from build123d import *

# Parameters (mm, degrees)
SKETCH1_R           = 55.5
BOSS_EXTRUDE1_DEPTH = 29.4
CUT_EXTRUDE1_DEPTH  = 19.4
SKETCH3_R           = 1.65
SKETCH3_R_2         = 2.8
CUT_EXTRUDE2_DEPTH  = 133.783969288
SKETCH4_R           = 11.3
CUT_EXTRUDE3_DEPTH  = 2
SKETCH5_R           = 3.3
CUT_EXTRUDE4_DEPTH  = 5
SKETCH6_R           = 40.3
SKETCH6_R_2         = 30.3
BOSS_EXTRUDE2_DEPTH = 59.8
BOSS_EXTRUDE3_DEPTH = 119.6
BOSS_EXTRUDE4_START = -29.4
BOSS_EXTRUDE4_DEPTH = 29.4
FILLET1_R           = 10
SKETCH9_W           = 2.2
SKETCH9_H           = 4.6
CUT_EXTRUDE5_DEPTH  = 11.5
SKETCH10_R          = 2.25
CUT_EXTRUDE6_DEPTH  = 8
SKETCH12_W          = 52.3
SKETCH12_H          = 55.486218433
SKETCH12_R          = 2.75
BOSS_EXTRUDE5_DEPTH = 10
SKETCH13_R          = 1.65
CUT_EXTRUDE7_DEPTH  = 240.292148847
SKETCH14_R          = 3.3
CUT_EXTRUDE8_DEPTH  = 6
SKETCH15_W          = 42.7
SKETCH15_H          = 42.7
CUT_EXTRUDE9_DEPTH  = 80
FILLET2_R           = 40
FILLET3_R           = 5
SKETCH16_R          = 2.25
CUT_EXTRUDE10_DEPTH = 4
SKETCH17_R          = 2.25
CUT_EXTRUDE11_DEPTH = 7
CUT_EXTRUDE14_DEPTH = 20
SKETCH20_R          = 11.25
CUT_EXTRUDE15_DEPTH = 2.2


with BuildPart() as part:
    # Sketch1 → Boss-Extrude1 (new body)
    with BuildSketch(Plane(origin=(0, 0, 0), x_dir=(1, 0, 0), z_dir=(0, 1, 0))):
        with BuildLine():
            Line((24.826614984, -60.071950097), (112.295843768, -23.922551543))
            ThreePointArc((112.295843768, -23.922551543), (113.643745306, -22.817703315), (114.15, -21.15))
            Line((114.15, -21.15), (114.15, 21.15))
            ThreePointArc((114.15, 21.15), (113.643745306, 22.817703315), (112.295843768, 23.922551543))
            Line((112.295843768, 23.922551543), (24.826614984, 60.071950097))
            ThreePointArc((24.826614984, 60.071950097), (-65, 0), (24.826614984, -60.071950097))
        make_face()
        with Locations(Location((0, 0, 0), (0, 0, 270))):
            Circle(SKETCH1_R, mode=Mode.SUBTRACT)
    extrude(amount=BOSS_EXTRUDE1_DEPTH)

    # Sketch2 → Cut-Extrude1 (cut)
    with BuildSketch(Plane(origin=(0, 29.4, 0), x_dir=(1, 0, 0), z_dir=(0, 1, 0))):
        with BuildLine():
            Line((69.5, 21.5), (110.5, 21.5))
            ThreePointArc((110.5, 21.5), (111.207106781, 21.207106781), (111.5, 20.5))
            Line((111.5, 20.5), (111.5, -20.5))
            ThreePointArc((111.5, -20.5), (111.207106781, -21.207106781), (110.5, -21.5))
            Line((110.5, -21.5), (69.5, -21.5))
            ThreePointArc((69.5, -21.5), (68.792893219, -21.207106781), (68.5, -20.5))
            Line((68.5, -20.5), (68.5, 20.5))
            ThreePointArc((68.5, 20.5), (68.792893219, 21.207106781), (69.5, 21.5))
        make_face()
    extrude(amount=-CUT_EXTRUDE1_DEPTH, mode=Mode.SUBTRACT)

    # Sketch3 → Cut-Extrude2 (cut, through all)
    with BuildSketch(Plane(origin=(0, 10, 0), x_dir=(1, 0, 0), z_dir=(0, 1, 0))):
        with Locations(Location((74.5, -15.5, 0), (0, 0, 270))):
            Circle(SKETCH3_R)
        with Locations(Location((105.5, -15.5, 0), (0, 0, 270))):
            Circle(SKETCH3_R)
        with Locations(Location((105.5, 15.5, 0), (0, 0, 270))):
            Circle(SKETCH3_R)
        with Locations(Location((74.5, 15.5, 0), (0, 0, 270))):
            Circle(SKETCH3_R)
        with Locations(Location((90, 0, 0), (0, 0, 270))):
            Circle(SKETCH3_R_2)
    extrude(amount=-CUT_EXTRUDE2_DEPTH, mode=Mode.SUBTRACT)

    # Sketch4 → Cut-Extrude3 (cut)
    with BuildSketch(Plane(origin=(0, 10, 0), x_dir=(1, 0, 0), z_dir=(0, 1, 0))):
        with Locations(Location((90, 0, 0), (0, 0, 270))):
            Circle(SKETCH4_R)
    extrude(amount=-CUT_EXTRUDE3_DEPTH, mode=Mode.SUBTRACT)

    # Sketch5 → Cut-Extrude4 (cut)
    with BuildSketch(Plane.XZ):
        with Locations(Location((74.5, 15.5, 0), (0, 0, 270))):
            Circle(SKETCH5_R)
        with Locations(Location((105.5, 15.5, 0), (0, 0, 270))):
            Circle(SKETCH5_R)
        with Locations(Location((74.5, -15.5, 0), (0, 0, 270))):
            Circle(SKETCH5_R)
        with Locations(Location((105.5, -15.5, 0), (0, 0, 270))):
            Circle(SKETCH5_R)
    extrude(amount=-CUT_EXTRUDE4_DEPTH, mode=Mode.SUBTRACT)



with BuildPart() as body_2:
    # Sketch6 → Boss-Extrude2 (new, symmetric)
    with BuildSketch(Plane.XY):
        with Locations((-120, 40.3)):
            Circle(SKETCH6_R)
        with Locations((-120, 40.3)):
            Circle(SKETCH6_R_2, mode=Mode.SUBTRACT)
    extrude(amount=BOSS_EXTRUDE2_DEPTH, both=True)

    # Sketch7 → Boss-Extrude3 (add)
    with BuildSketch(Plane.XY.offset(59.8)):
        with BuildLine():
            Line((-65, 29.4), (-65, 0))
            Line((-65, 0), (-120, 0))
            ThreePointArc((-120, 0), (-95.660525889, 8.18022416), (-81.20206191, 29.4))
            Line((-81.20206191, 29.4), (-65, 29.4))
        make_face()
    extrude(amount=-BOSS_EXTRUDE3_DEPTH)


with BuildPart() as part_1:
    add(part.part)

    add(body_2.part)  # Boss-Extrude4 merges body 2
    # Sketch8 → Boss-Extrude4 (add)
    with BuildSketch(Plane(origin=(0, 29.4, 0), x_dir=(1, 0, 0), z_dir=(0, 1, 0)).offset(BOSS_EXTRUDE4_START)):
        with BuildLine():
            ThreePointArc((-25.474693325, -59.8), (-54.225709183, -35.840932794), (-65, 1.13e-07))
            Line((-65, 1.13e-07), (-65, -59.8))
            Line((-65, -59.8), (-25.474693325, -59.8))
        make_face()
        with BuildLine():
            Line((-25.474693325, 59.8), (-65, 59.8))
            Line((-65, 59.8), (-65, 1.13e-07))
            ThreePointArc((-65, 1.13e-07), (-54.225709121, 35.840932889), (-25.474693325, 59.8))
        make_face()
    extrude(amount=BOSS_EXTRUDE4_DEPTH)

    # Fillet1
    fillet1_edges = [part_1.edges().sort_by_distance(p)[0] for p in [
        (-81.20206191, 29.4, 0),
    ]]
    fillet(fillet1_edges, radius=FILLET1_R)

    # Sketch9 → Cut-Extrude5 (cut)
    with BuildSketch(Plane(origin=(0, 29.4, 0), x_dir=(1, 0, 0), z_dir=(0, 1, 0))):
        with Locations((66.4, 0)):
            Rectangle(SKETCH9_W, SKETCH9_H)
    extrude(amount=-CUT_EXTRUDE5_DEPTH, mode=Mode.SUBTRACT)

    # Sketch10 → Cut-Extrude6 (cut)
    with BuildSketch(Plane(origin=(0, 29.4, 0), x_dir=(1, 0, 0), z_dir=(0, 1, 0))):
        with Locations(Location((90, -27.612605503, 0), (0, 0, 270))):
            Circle(SKETCH10_R)
        with Locations(Location((90, 27.387394497, 0), (0, 0, 270))):
            Circle(SKETCH10_R)
    extrude(amount=-CUT_EXTRUDE6_DEPTH, mode=Mode.SUBTRACT)

    # Sketch12 → Boss-Extrude5 (add)
    with BuildSketch(Plane(origin=(0, 0, -59.8), x_dir=(-1, 0, 0), z_dir=(0, 0, -1))):
        with Locations((120, 98.706890784)):
            Rectangle(SKETCH12_W, SKETCH12_H)
        with Locations((120, 100.3)):
            Circle(SKETCH12_R, mode=Mode.SUBTRACT)
    extrude(amount=-BOSS_EXTRUDE5_DEPTH)

    # Sketch13 → Cut-Extrude7 (cut, through all)
    with BuildSketch(Plane(origin=(0, 0, -59.8), x_dir=(-1, 0, 0), z_dir=(0, 0, -1))):
        with Locations((104.5, 115.8)):
            Circle(SKETCH13_R)
        with Locations((104.5, 84.8)):
            Circle(SKETCH13_R)
        with Locations((135.5, 84.8)):
            Circle(SKETCH13_R)
        with Locations((135.5, 115.8)):
            Circle(SKETCH13_R)
    extrude(amount=-CUT_EXTRUDE7_DEPTH, mode=Mode.SUBTRACT)

    # Sketch14 → Cut-Extrude8 (cut)
    with BuildSketch(Plane(origin=(0, 0, -59.8), x_dir=(-1, 0, 0), z_dir=(0, 0, -1))):
        with Locations((104.5, 115.8)):
            Circle(SKETCH14_R)
        with Locations((104.5, 84.8)):
            Circle(SKETCH14_R)
        with Locations((135.5, 84.8)):
            Circle(SKETCH14_R)
        with Locations((135.5, 115.8)):
            Circle(SKETCH14_R)
    extrude(amount=-CUT_EXTRUDE8_DEPTH, mode=Mode.SUBTRACT)

    # Sketch15 → Cut-Extrude9 (cut)
    with BuildSketch(Plane.XY.offset(-49.8)):
        with Locations((-120, 100.3)):
            Rectangle(SKETCH15_W, SKETCH15_H)
    extrude(amount=CUT_EXTRUDE9_DEPTH, mode=Mode.SUBTRACT)

    # Fillet2
    fillet2_edges = [part_1.edges().sort_by_distance(p)[0] for p in [
        (-93.85, 70.963781567, -54.8),
        (-146.15, 70.963781567, -54.8),
    ]]
    fillet(fillet2_edges, radius=FILLET2_R)

    # Fillet3
    fillet3_edges = [part_1.edges().sort_by_distance(p)[0] for p in [
        (-93.85, 126.45, -54.8),
        (-146.15, 126.45, -54.8),
    ]]
    fillet(fillet3_edges, radius=FILLET3_R)

    # Sketch16 → Cut-Extrude10 (cut)
    with BuildSketch(Plane.XY.offset(-49.8)):
        with Locations((-143, 77.3)):
            Circle(SKETCH16_R)
        with Locations((-97, 77.3)):
            Circle(SKETCH16_R)
    extrude(amount=-CUT_EXTRUDE10_DEPTH, mode=Mode.SUBTRACT)

    # Sketch17 → Cut-Extrude11 (cut)
    with BuildSketch(Plane(origin=(0, 78.95, 0), x_dir=(1, 0, 0), z_dir=(0, 1, 0))):
        with Locations(Location((-120, -25.2, 0), (0, 0, 270))):
            Circle(SKETCH17_R)
    extrude(amount=-CUT_EXTRUDE11_DEPTH, mode=Mode.SUBTRACT)

    # Sketch18 → Cut-Extrude14 (cut)
    with BuildSketch(Plane.XY.offset(59.8)):
        Polygon((-122.3, 7), (-117.7, 7), (-117.7, 4.8), (-115, 4.8), (-114, 3.8), (-114, 2.8), (-115, 1.8), (-115, 0), (-125, 0), (-125, 1.8), (-126, 2.8), (-126, 3.8), (-125, 4.8), (-122.3, 4.8), align=None)
    extrude(amount=-CUT_EXTRUDE14_DEPTH, mode=Mode.SUBTRACT)

    # Sketch20 → Cut-Extrude15 (cut)
    with BuildSketch(Plane.XY.offset(-49.8)):
        with Locations((-120, 100.3)):
            Circle(SKETCH20_R)
    extrude(amount=-CUT_EXTRUDE15_DEPTH, mode=Mode.SUBTRACT)


solid = part_1.part
Check sheet for the modelled part. Datum: model origin and axes. Units: mm. A direction names the side the tool comes from. Round coordinates to 2 decimals unless told otherwise and drop trailing zeros. Loops run counter-clockwise (first coordinate to the right, second up) from the corner with the lowest first, then second, coordinate; pieces in that order, holes last. Notation, with made-up numbers: (-38.75, -18) -> (-5.75, -18) arc R23 cw to (-5.75, 15) -> close; hole circle Ø9 at (4, 36.5). An arc over 180 degrees is marked (long way). Put each result on its own line as item: value. Start each with the question number.
1. Scan lines: probe 1 along X at (y, z) = (82.5, -54.5); probe 2 along X at (y, z) = (77, -52); probe 3 along Y at (x, z) = (-104.5, -51.55). Record each from-to range of solid material in increasing order.
2. Draft check along X on faces 5 (the face through (67.95, 14.49, 42.25)), 6 (the face through (-92, 64, -59.8)), 7 (the face through (-134, 86, -53.8)), 8 (the face through (-101.2, 84.9, -56.8)). Enter one of: +X half, -X half, draft (parallel to the pull), parting line (faces both ways), or undercut.
3. Gauge pin test, flat ends, axial feed: pin 1 (4 mm diameter, centred on x = -120, z = 25.2, fed in from +Y); pin 2 (12 mm diameter, centred on x = -102, y = 49.5, fed in from -Z); pin 3 (1.4 mm diameter, centred on x = -119, z = 49, fed in from -Y); pin 4 (2.5 mm diameter, centred on y = 5.5, z = 46.5, fed in from +X). Record the tip position at first contact, or that the pin passes through.
4. Section check A-A (y = 67.5). Enter the section's corners in (x, z), plus the area to 3 significant figures.
5. Access from +Z, -Z, +X, -X, +Y, -Y to the whole of each face (thin tool, end or side, straight path). Record for faces 1 (the face through (-118, 98, -52)), 2 (the face through (-146.15, 103, -55)), 3 (the face through (-133.07, 87.03, -56.84)), 4 (the face through (107.73, 2.46, -13.07)).
6. Section check B-B (x = -60). Enter the section's corners in (y, z).
7. Section check C-C (y = 48). Enter the section's corners in (x, z), plus the area to 3 significant figures.
Findings:
1. probe 1: x = -146.29 to -137.87, -133.13 to -106.87, -102.13 to -93.71
1. probe 2: x = -147.14 to -145.23, -140.77 to -99.23, -94.77 to -92.86
1. probe 3: y = 0 to 14.26, 66.34 to 83.15, 86.45 to 114.15, 117.45 to 126.45
2. face 5: +X half
2. face 6: draft
2. face 7: undercut
2. face 8: undercut
3. pin 1: stops at y = 71.95
3. pin 2: passes through
3. pin 3: stops at y = 7
3. pin 4: stops at x = 60.69
4. outline: (-150.59, -59.8) -> (-133.35, -59.8) -> (-133.35, 59.8) -> (-149.74, 59.8) -> (-149.74, -49.8) -> (-150.59, -49.8) -> close; (-106.65, -59.8) -> (-89.41, -59.8) -> (-89.41, -49.8) -> (-90.26, -49.8) -> (-90.26, 59.8) -> (-106.65, 59.8) -> close
4. area: 3,940 mm^2
5. face 1: +Z
5. face 2: +Z, -Z, -X, +Y
5. face 3: -Z
5. face 4: -Y
6. outline: (0, -59.8) -> (29.4, -59.8) -> (29.4, 59.8) -> (0, 59.8) -> close
7. outline: (-159.56, -59.8) -> (-149.31, -59.8) -> (-149.31, 59.8) -> (-159.56, 59.8) -> close; (-90.69, -59.8) -> (-80.44, -59.8) -> (-80.44, 59.8) -> (-90.69, 59.8) -> close
7. area: 2,450 mm^2
